```python
from build123d import *

# Parameters (mm, degrees)
F1_DEPTH = 125.25
F2_W     = 55.821885
F2_H     = 5.25
F3_DEPTH = 3
F4_R     = 2.5
F5_DEPTH = 25


with BuildPart() as f1:
    # F0 (on Front) → F1 (new body)
    with BuildSketch(Plane.XZ):
        Polygon((0, 3.79), (0, 0), (15.67, 0), (15.67, 3.79), (18.435, 6.555), (15.67, 9.32), (0, 9.32), (-2.765, 6.555), align=None)
    extrude(amount=F1_DEPTH)

    # F2 (on face) → F3 (cut)
    with BuildSketch(Plane.XY.offset(9.32)):
        with Locations((8.211463, -17.625)):
            Rectangle(F2_W, F2_H)
        with Locations((8.211463, -27.625)):
            Rectangle(F2_W, F2_H)
        with Locations((8.211463, -37.625)):
            Rectangle(F2_W, F2_H)
        with Locations((8.211463, -47.625)):
            Rectangle(F2_W, F2_H)
        with Locations((8.211463, -57.625)):
            Rectangle(F2_W, F2_H)
        with Locations((8.211463, -67.625)):
            Rectangle(F2_W, F2_H)
        with Locations((8.211463, -77.625)):
            Rectangle(F2_W, F2_H)
        with Locations((8.211463, -87.625)):
            Rectangle(F2_W, F2_H)
        with Locations((8.211463, -97.625)):
            Rectangle(F2_W, F2_H)
        with Locations((8.211463, -107.625)):
            Rectangle(F2_W, F2_H)
    extrude(amount=-F3_DEPTH, mode=Mode.SUBTRACT)

    # F4 (on face) → F5 (cut)
    with BuildSketch(Plane.XY.offset(9.32)):
        with Locations((7.835, -7.5)):
            Circle(F4_R)
        with Locations((7.835, -117.75)):
            Circle(F4_R)
    extrude(amount=-F5_DEPTH, mode=Mode.SUBTRACT)


solid = f1.part
```
Check sheet for the modelled part. Datum: model origin and axes. Units: mm. A direction names the side the tool comes from. Round coordinates to 2 decimals unless told otherwise and drop trailing zeros. Write each loop counter-clockwise with the first axis right and the second up, starting at its lowest first coordinate (ties: lowest second). Pieces come first, ordered by that corner, then holes. Notation, with made-up numbers: M -29,3.25 L 22,3.25 A34 cw 22,38.25 Z; hole C 53.25,44.5 d7. An arc over 180 degrees is marked long. Write item = value, one per line. Start each with the question number.
1. Release check for a two-part mould opening along Y. For faces 3 (the flat face through (8, -75, 8)), 4 (the flat face through (17.07, -62.59, 7.92)) record: pulls with the +Y half, pulls with the -Y half, needs draft (parallel to the pull), parting line crosses it, or undercut.
2. Section check A-A, the plane y = -117.75. Record the cut outline in (x, z) (3 decimals), then the cut area to 3 significant figures.
3. Section check C-C, the plane y = -78. Record the cut outline in (x, z), then the cut area to 3 significant figures.
4. Scan lines: line 1 (Y direction, x = 7.5, z = 1.5); line 2 (Y direction, x = 9, z = 4.25); line 3 (X direction, y = -99.5, z = 3). Record each from-to range of solid material in increasing order. Write a range as [from, to].
5. Section check D-D, the plane x = 6.5. State how many separate pieces and enclosed holes the cut face has, then the cut area to 3 significant figures.
6. Section check B-B, the plane z = 1.5. Record the cut outline in (x, y) (3 decimals).
7. Tool access check on faces 1 (the flat face through (-1.4, -61.75, 5.19)), 2 (the flat face through (8, -60.25, 8)). Record the directions out of +Z, -Z, +X, -X, +Y, -Y that give a thin tool (end or side, any length) a straight path to the whole face; none if there is none.
8. Gauge pin test, flat ends, axial feed: pin 1 (1.9 mm diameter, centred on y = -32, z = 1, fed in from +X); pin 2 (2.5 mm diameter, centred on x = 12, y = -37, fed in from +Z); pin 3 (3 mm diameter, centred on y = -14.5, z = 2.5, fed in from +X). Record the tip position at first contact, or that the pin passes through.
Results found:
q1.face_3 = undercut
q1.face_4 = needs draft
q2.outline = M -2.765,6.555 L 0,3.79 L 0,0 L 5.335,0 L 5.335,9.32 L 0,9.32 Z; M 10.335,0 L 15.67,0 L 15.67,3.79 L 18.435,6.555 L 15.67,9.32 L 10.335,9.32 Z
q2.area = 115 mm^2
q3.outline = M -2.53,6.32 L 0,3.79 L 0,0 L 15.67,0 L 15.67,3.79 L 18.2,6.32 Z
q3.area = 105 mm^2
q4.line_1 = [-125.25, -120.23], [-115.27, -9.98], [-5.02, 0]
q4.line_2 = [-125.25, -119.96], [-115.54, -9.71], [-5.29, 0]
q4.line_3 = [0, 15.67]
q5.separate_pieces = 3
q5.enclosed_holes = 0
q5.area = 931 mm^2
q6.outline = M 0,-125.25 L 15.67,-125.25 L 15.67,0 L 0,0 Z; hole C 7.835,-117.75 d5; hole C 7.835,-7.5 d5
q7.face_1 = -Z, -X, +Y, -Y
q7.face_2 = +Z, +X, -X
q8.pin_1 = 15.67
q8.pin_2 = 6.32
q8.pin_3 = 15.88
